Source: CAD feature listing. Evaluate the final solid. Frame: model axes, mm. Face numbers are marked on the shaded views. Give positions to 0.01 mm unless a question says otherwise; leave off trailing zeros. Write each loop counter-clockwise with the first axis right and the second up, starting at its lowest first coordinate (ties: lowest second). Pieces come first, ordered by that corner, then holes. Notation, with made-up numbers: (59.25, 11.25) -> (75.25, 11.25) arc R29 cw to (75.25, 41.25) -> close; hole circle Ø8 at (-15.5, 31). An arc over 180 degrees is marked (long way). Answer as a JSON object with one key per item and string values. Group by question number.
Item 1: Section query A-A on y = -20.25. Return the cut outline in (x, z), plus the area to 3 significant figures.
Item 2: Pull-direction query (Z, two-part tool) for the marked faces 1, 2 and 3; classes: pulls with the +Z half, pulls with the -Z half, needs draft (parallel to the pull), parting line crosses it, or undercut.
Item 3: Ray query, probe 1 along Z at (x, y) = (-138, -11.25); probe 2 along X at (y, z) = (-21, -100); probe 3 along Z at (x, y) = (-178, -19) (3 decimals). Return the intervals inside material, ascending. Write a range as from..to.
Item 4: First-contact query: pin 1 Ø1 at (x, z) = (-185, -100.5) entering from +Y. Flat tip, straight axial feed; report the tip coordinate or a pass-through.
Item 5: Section query B-B on y = -5.25. Return the cut outline in (x, z).
from build123d import *

# Parameters (mm, degrees)
F0_W     = 123.2844814658
F0_H     = 132.5032711029
F1_DEPTH = 25.4
F2_R     = 33.9258484302
F3_DEPTH = 25.4
F3_TAPER = -3


with BuildPart() as f1:
    # F0 (on Front) → F1 (new body)
    with BuildSketch(Plane.XZ):
        with Locations((-162.3135991395, -66.2516355515)):
            Rectangle(F0_W, F0_H)
    extrude(amount=F1_DEPTH)

    # F2 (on face) → F3 (cut)
    with BuildSketch(Plane.XZ.offset(25.4)):
        with Locations((-159.5336198807, -69.13626194)):
            Circle(F2_R)
    extrude(amount=-F3_DEPTH, taper=F3_TAPER, mode=Mode.SUBTRACT)


solid = f1.part
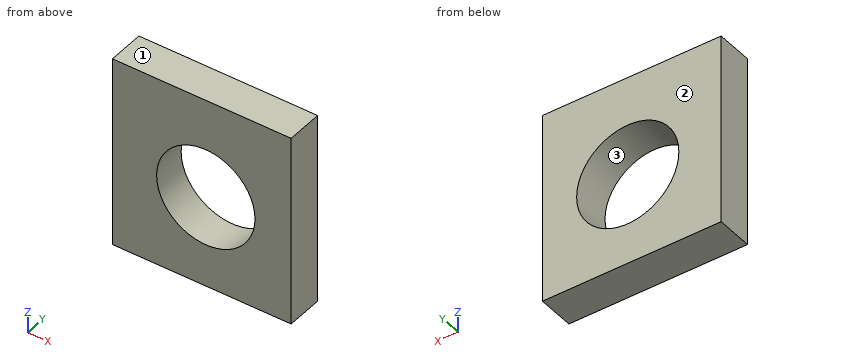
Worked answers:
{
 "1": {"outline": "(-223.96, -132.5) -> (-100.67, -132.5) -> (-100.67, 0) -> (-223.96, 0) -> close; hole circle Ø68.39 at (-159.53, -69.14)", "area": "12,700 mm^2"},
 "2": {"face 1": "pulls with the +Z half", "face 2": "needs draft", "face 3": "undercut"},
 "3": {"probe 1": "-132.5..-96.3, -41.97..0", "probe 2": "-223.96..-174.17, -144.9..-100.67", "probe 3": "-132.503..-97.995, -40.278..0"},
 "4": {"pin 1": "y = 0"},
 "5": {"outline": "(-223.96, -132.5) -> (-100.67, -132.5) -> (-100.67, 0) -> (-223.96, 0) -> close; hole circle Ø69.96 at (-159.53, -69.14)"}
}
